```python
from build123d import *

# Parameters (mm, degrees)
F0_W     = 4
F0_H     = 99
F0_H_2   = 4
F0_W_2   = 166
F1_DEPTH = 1


with BuildPart() as f1:
    # F0 (on Front) → F1 (new body, symmetric)
    with BuildSketch(Plane.XZ):
        with Locations((-85, 2)):
            Rectangle(F0_W, F0_H)
        with Locations((-85, -49.5)):
            Rectangle(F0_W, F0_H_2)
        with Locations((0, -49.5)):
            Rectangle(F0_W_2, F0_H_2)
        with Locations((85, 2)):
            Rectangle(F0_W, F0_H)
        with Locations((85, -49.5)):
            Rectangle(F0_W, F0_H_2)
    extrude(amount=F1_DEPTH, both=True)


solid = f1.part
```
Geometry check sheet. Reference: the model listing, model coordinates, mm. Coordinates: 2 decimals unless noted, no trailing zeros. Order: outer loops, then holes, each group sorted by start corner. A loop starts at its lowest first (then second) coordinate and runs counter-clockwise, first axis right, second up. Notation, with made-up numbers: (37, 53) - (80, 53) arc R29 cw to (80, 85) - close; hole circle Ø9 at (-30, -34). An arc over 180 degrees is marked (long way). Answer as a JSON object with one key per item and string values. Group by question number.
Item 1: Sectioned sample at C-C, the plane x = -6.5. Record the cut outline in (y, z).
Item 2: Sectioned sample at B-B, the plane y = 0.45. Record the cut outline in (x, z), and give its area (3 significant figures).
Item 3: Sectioned sample at A-A, the plane z = 36. Record the cut outline in (x, y), and give its area (3 significant figures).
Item 4: Scan lines: probe 1 along X at (y, z) = (0.05, 9.5); probe 2 along Z at (x, y) = (25.5, -0.6). Record each from-to range of solid material in increasing order.
Item 5: Depth check by flat-ended pin: pin 1 Ø1 at (x, y) = (4, 0.5) entering from +Z. Enter the tip coordinate at first touch or a pass-through.
Resolved:
{
 "1": {"outline": "(-1, -51.5) - (1, -51.5) - (1, -47.5) - (-1, -47.5) - close"},
 "2": {"outline": "(-87, -51.5) - (87, -51.5) - (87, 51.5) - (83, 51.5) - (83, -47.5) - (-83, -47.5) - (-83, 51.5) - (-87, 51.5) - close", "area": "1,490 mm^2"},
 "3": {"outline": "(-87, -1) - (-83, -1) - (-83, 1) - (-87, 1) - close; (83, -1) - (87, -1) - (87, 1) - (83, 1) - close", "area": "16.0 mm^2"},
 "4": {"probe 1": "-87 to -83, 83 to 87", "probe 2": "-51.5 to -47.5"},
 "5": {"pin 1": "z = -47.5"}
}
